Part model, mm, in its own coordinate system. Give positions to 0.01 mm unless a question says otherwise; leave off trailing zeros. Loops run counter-clockwise (first coordinate to the right, second up) from the corner with the lowest first, then second, coordinate; pieces in that order, holes last. Notation, with made-up numbers: (-31.75, -15.75) -> (12.25, -15.75) arc R31 cw to (12.25, 12.25) -> close; hole circle Ø11 at (-10, 39). An arc over 180 degrees is marked (long way). One line per question, with ' | ' between items.
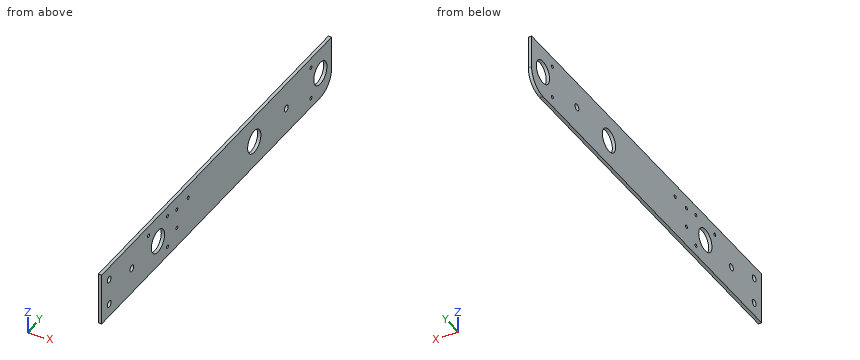
Autodesk Inventor part; units mm, degrees
ref_plane "YZ Plane" through (0, 0, 0) normal (1, 0, 0) x (0, 1, 0)
ref_plane "XZ Plane" through (0, 0, 0) normal (0, 1, 0) x (-1, 0, 0)
ref_plane "XY Plane" through (0, 0, 0) normal (0, 0, 1) x (1, 0, 0)
sketch "Sketch1" plane through (0, 0, 0) normal (1, 0, 0) x (0, 1, 0)
  line L0 (386.842, -25.4) -> (0, -25.4) construction
  circle A0 centre (94.742, -25.4) radius 11.1125
  circle A1 centre (367.792, -25.4) radius 11.1125
  circle A2 centre (256.667, -25.4) radius 11.1125
  circle A3 centre (310.642, -25.4) radius 3.175
  line L1 (0, 0) -> (386.842, 0)
  line L2 (386.842, 0) -> (386.842, -50.8)
  line L3 (386.842, -50.8) -> (0, -50.8)
  line L4 (0, -50.8) -> (0, 0)
  line L5 (78.867, -9.525) -> (110.617, -9.525) construction
  line L6 (110.617, -9.525) -> (110.617, -41.275) construction
  circle A4 centre (110.617, -9.525) radius 1.5875
  circle A5 centre (110.617, -41.275) radius 1.5875
  circle A6 centre (78.867, -9.525) radius 1.5875
  line L7 (351.917, -9.525) -> (351.917, -41.275) construction
  circle A7 centre (351.917, -41.275) radius 1.5875
  circle A8 centre (351.917, -9.525) radius 1.5875
  line L8 (12.7, -50.8) -> (12.7, 0) construction
  circle A9 centre (12.7, -38.1) radius 3.175
  circle A10 centre (12.7, -12.7) radius 3.175
  line L9 (126.492, 0) -> (126.492, -50.8) construction
  line L10 (126.492, -12.7) -> (145.542, -12.7) construction
  circle A11 centre (126.492, -12.7) radius 1.5875
  circle A12 centre (145.542, -12.7) radius 1.5875
  circle A13 centre (126.492, -31.75) radius 1.5875
  circle A14 centre (50.8, -25.4) radius 3.175
  point P0 (351.917, -25.4)
  dimension "d3" = 22.225
  dimension "d4" = 273.05
  dimension "d9" = 161.925
  dimension "d12" = 6.35
  dimension "d13" = 57.15
  dimension "d15" = 50.8
  dimension "d16" = 19.05
  dimension "d17" = 94.742
  dimension "d18" = 3.175
  dimension "d19" = 9.525
  dimension "d20" = 31.75
  dimension "d22" = 15.875
  dimension "d23" = 3.175
  dimension "d24" = 15.875
  dimension "d25" = 31.75
  dimension "d26" = 6.35
  dimension "d27" = 12.7
  dimension "d28" = 25.4
  dimension "d29" = 19.05
  dimension "d30" = 19.05
  dimension "d31" = 6.35
  dimension "d32" = 31.75
  dimension "d33" = 38.1
extrude "Extrusion1" add sketch "Sketch1" along normal blind 3.175
fillet "Fillet1" radius 19.05 1 edges at (1.5875, 386.842, -50.8)
equation "\"d30\" = d29"
properties part number "Back Plate"
1) Saw through at B-B (y = 50.8). Give the cut face in (x, z) (3 decimals), and give its area (3 significant figures).
Found:
outline: (0, -50.8) -> (3.175, -50.8) -> (3.175, -28.575) -> (0, -28.575) -> close; (0, -22.225) -> (3.175, -22.225) -> (3.175, 0) -> (0, 0) -> close | area: 141 mm2
2) Saw through at C-C (z = -25.4). Give the cut face in (x, y) (1 decimal).
Found:
outline: (0, 0) -> (3.2, 0) -> (3.2, 47.6) -> (0, 47.6) -> close; (0, 54) -> (3.2, 54) -> (3.2, 83.6) -> (0, 83.6) -> close; (0, 105.9) -> (3.2, 105.9) -> (3.2, 245.6) -> (0, 245.6) -> close; (0, 267.8) -> (3.2, 267.8) -> (3.2, 307.5) -> (0, 307.5) -> close; (0, 313.8) -> (3.2, 313.8) -> (3.2, 356.7) -> (0, 356.7) -> close; (0, 378.9) -> (3.2, 378.9) -> (3.2, 386.8) -> (0, 386.8) -> close
3) Saw through at A-A (x = 1.5). State how many separate pieces and enclosed holes the cut face has, and give its area (3 significant figures).
Found:
separate pieces: 1 | enclosed holes: 15 | area: 18,200 mm2
4) Drill centre lines: line 1 (Z direction, x = 1.35, y = 12.7) (3 decimals); line 2 (Y direction, x = 1.85, z = -34.5); line 3 (Y direction, x = 2.7, z = -33). Where is each one in solid material? Low to high.
Found:
line 1: -50.8 to -41.275, -34.925 to -15.875, -9.525 to 0 | line 2: 0 to 88.36, 101.12 to 250.29, 263.04 to 361.41, 374.17 to 386.64 | line 3: 0 to 86.63, 102.85 to 125.51, 127.47 to 248.56, 264.77 to 359.68, 375.9 to 386.8
